For this review, take the finished solid that the model builds, in its own axes (mm). A direction names the side the tool comes from. Coordinates: 2 decimals unless noted, no trailing zeros. Order: outer loops, then holes, each group sorted by start corner. A loop starts at its lowest first (then second) coordinate and runs counter-clockwise, first axis right, second up.
from build123d import *

# Parameters (mm, degrees)
SKETCH1_W                 = 6.35
SKETCH1_H                 = 38.1
SKETCH1_W_2               = 12.7
SKETCH1_H_2               = 6.35
BOSS_EXTRUDE1_DEPTH       = 12.7
F_5_0MM_DOWEL_HOLE1_D     = 5.25
F_5_0MM_DOWEL_HOLE1_DEPTH = 9.906
F_5_0MM_DOWEL_HOLE1_TIP   = 1.577259125
F_5_0MM_DOWEL_HOLE2_D     = 5.25
F_5_0MM_DOWEL_HOLE2_DEPTH = 9.906
F_5_0MM_DOWEL_HOLE2_TIP   = 1.577259125


with BuildPart() as part:
    # Sketch1 → Boss-Extrude1 (new body)
    with BuildSketch(Plane(origin=(0, 0, 0), x_dir=(1, 0, 0), z_dir=(0, 1, 0))):
        with Locations((3.175, 19.05)):
            Rectangle(SKETCH1_W, SKETCH1_H)
        with Locations((12.7, 3.175)):
            Rectangle(SKETCH1_W_2, SKETCH1_H_2)
    extrude(amount=BOSS_EXTRUDE1_DEPTH)

    # Ø5.0mm Dowel Hole1
    with Locations(Plane.ZY):
        with Locations((-31.75, 6.35), (-19.05, 6.35)):
            Hole(F_5_0MM_DOWEL_HOLE1_D / 2, depth=F_5_0MM_DOWEL_HOLE1_DEPTH)
            with Locations((0, 0, -(F_5_0MM_DOWEL_HOLE1_DEPTH + F_5_0MM_DOWEL_HOLE1_TIP / 2))):  # 118° drill point
                Cone(0, F_5_0MM_DOWEL_HOLE1_D / 2, F_5_0MM_DOWEL_HOLE1_TIP, mode=Mode.SUBTRACT)

    # Ø5.0mm Dowel Hole2
    with Locations(Plane(origin=(0, 0, -6.35), x_dir=(-1, 0, 0), z_dir=(0, 0, -1))):
        with Locations((-12.7, 6.35)):
            Hole(F_5_0MM_DOWEL_HOLE2_D / 2, depth=F_5_0MM_DOWEL_HOLE2_DEPTH)
            with Locations((0, 0, -(F_5_0MM_DOWEL_HOLE2_DEPTH + F_5_0MM_DOWEL_HOLE2_TIP / 2))):  # 118° drill point
                Cone(0, F_5_0MM_DOWEL_HOLE2_D / 2, F_5_0MM_DOWEL_HOLE2_TIP, mode=Mode.SUBTRACT)


solid = part.part
1. The part is to be moulded in two halves that separate along Z. For faces 3 (the face through (5, 12.7, -15)), 4 (the face through (9, 6, 0)), 5 (the face through (3.22, 4.75, -29.67)), 6 (the face through (3, 6, -38.1)), say which applies: +Z half, -Z half, draft (parallel to the pull), parting line (faces both ways), or undercut.
Answer below:
face 3: draft
face 4: +Z half
face 5: undercut
face 6: -Z half
2. Take a section at D-D, the plane z = -4. Give the boundary of the cut face in (x, y) (3 decimals), plus the area to 3 significant figures.
Answer below:
outline: (0, 0) - (19.05, 0) - (19.05, 12.7) - (0, 12.7) - close; hole circle Ø5.25 at (12.7, 6.35)
area: 220 mm2
3. Take a section at C-C, the plane y = 6.35. Give the boundary of the cut face in (x, z) (3 decimals).
Answer below:
outline: (0, -38.1) - (6.35, -38.1) - (6.35, -34.375) - (0, -34.375) - close; (0, -29.125) - (6.35, -29.125) - (6.35, -21.675) - (0, -21.675) - close; (0, -16.425) - (6.35, -16.425) - (6.35, -6.35) - (10.075, -6.35) - (10.075, 0) - (0, 0) - close; (15.325, -6.35) - (19.05, -6.35) - (19.05, 0) - (15.325, 0) - close
4. Take a section at A-A, the plane z = -31.75. Give the boundary of the cut face in (x, y) (3 decimals).
Answer below:
outline: (0, 0) - (6.35, 0) - (6.35, 3.725) - (0, 3.725) - close; (0, 8.975) - (6.35, 8.975) - (6.35, 12.7) - (0, 12.7) - close
5. Take a section at B-B, the plane x = 12.7. Give the boundary of the cut face in (y, z) (3 decimals).
Answer below:
outline: (0, -6.35) - (3.725, -6.35) - (3.725, 0) - (0, 0) - close; (8.975, -6.35) - (12.7, -6.35) - (12.7, 0) - (8.975, 0) - close
6. Clearance check with flat-ended pins moving along their axes: pin 1 Ø6.5 at (y, z) = (5.5, -29) entering from +X; pin 2 Ø6 at (x, y) = (16, 9) entering from -Z. State where each tip first meets the part, or that it passes through.
Answer below:
pin 1: stops at x = 6.35
pin 2: stops at z = -6.35
7. To check wall thickness, follow L1, parallel to Y at x = 2.25, z = -19.05 (3 decimals); L2, parallel to Z at x = 2.5, y = 5.75; L3, parallel to Z at x = 3.5, y = 4. State the ranges of each line that lie inside material, in increasing order.
Answer below:
L1: y = 0 to 3.725, 8.975 to 12.7
L2: z = -38.1 to -34.31, -29.19 to -21.61, -16.49 to 0
L3: z = -38.1 to -32.92, -30.58 to -20.22, -17.88 to 0
8. Machinability: for faces 1 (the face through (19.05, 6, -3)), 2 (the face through (13, 3, -6.35)), which of the approach directions +Z, -Z, +X, -X, +Y, -Y give a long, thin tool a straight path to every point of the face, cutting with its end or side? Answer none if there is none.
Answer below:
face 1: +Z, -Z, +X, +Y, -Y
face 2: -Z, +X, +Y, -Y
